Geometry: final body of the model. Coordinates: model frame, mm. A direction names the side the tool comes from. Round coordinates to 2 decimals unless told otherwise and drop trailing zeros. Write each loop counter-clockwise with the first axis right and the second up, starting at its lowest first coordinate (ties: lowest second). Pieces come first, ordered by that corner, then holes. Notation, with made-up numbers: (68, 85.25) -> (81, 85.25) arc R28 ccw to (81, 122.25) -> close; hole circle Ø5 at (44.25, 50). An arc over 180 degrees is marked (long way). One line per item, written item: value. Start each with the question number.
from build123d import *

# Parameters (mm, degrees)
F1_DEPTH = 10
F2_DEPTH = 85
F3_W     = 20
F3_H     = 25
F4_DEPTH = 88.4


with BuildPart() as f1:
    # F0 (on Top) → F1 (new body)
    with BuildSketch(Plane.XY):
        Polygon((-180, 30), (-180, 0), (0, 0), (0, 30), (-10, 30), (-10, 10), (-170, 10), (-170, 30), align=None)
    extrude(amount=F1_DEPTH)

    # F1_face (on face) → F2 (join)
    with BuildSketch(Plane(origin=(-90, 7.727273, 10), x_dir=(1, 0, 0), z_dir=(0, 0, 1))):
        Polygon((-90, 22.272727), (-90, -7.727273), (90, -7.727273), (90, 22.272727), (80, 22.272727), (80, 2.272727), (-80, 2.272727), (-80, 22.272727), align=None)
    extrude(amount=-F2_DEPTH)

    # F3 (on face) → F4 (cut)
    with BuildSketch(Plane.YZ):
        with Locations((20, -32.5)):
            Rectangle(F3_W, F3_H)
    extrude(amount=-F4_DEPTH, mode=Mode.SUBTRACT)


solid = f1.part
(1) Line query: probe 1 along X at (y, z) = (20.5, -63); probe 2 along Y at (x, z) = (-83, -63); probe 3 along X at (y, z) = (17, -38.5). Output: solid intervals per line, ascending.
(2) Section query A-A (y = 18.75). Output: boundary loops of the cut face in (x, z).
(3) Pull-direction query (Z, two-part tool) for faces 3 (the face through (-5, 20, -20)), 4 (the face through (-10, 20, -5)), 5 (the face through (-5, 20, -45)), 6 (the face through (-111, 9, 10)); classes: pulls with the +Z half, pulls with the -Z half, needs draft (parallel to the pull), parting line crosses it, or undercut.
(4) Section query C-C (x = -154.5). Output: boundary loops of the cut face in (y, z).
(5) Section query B-B (z = -49.5). Output: boundary loops of the cut face in (x, y).
(6) Set-up query: faces 1 (the face through (0, 8, -32)), 2 (the face through (-10, 20, -60)). Return all of +Z, -Z, +X, -X, +Y, -Y with unobstructed straight access to the full face (end or side cutting, diameter ignored); none if empty.
(7) Pin query (flat end, axial travel): pin 1 (2 mm diameter, centred on x = -83.5, z = -59.5, fed in from +Y). Return the tip coordinate at first contact, or that it passes through.
(8) Section query D-D (z = -31.5). Output: boundary loops of the cut face in (x, y), and give its area (3 significant figures).
Results list:
1. probe 1: x = -180 to -170, -10 to 0
1. probe 2: y = 0 to 10
1. probe 3: x = -180 to -170
2. outline: (-180, -75) -> (-170, -75) -> (-170, 10) -> (-180, 10) -> close; (-10, -75) -> (0, -75) -> (0, -45) -> (-10, -45) -> close; (-10, -20) -> (0, -20) -> (0, 10) -> (-10, 10) -> close
3. face 3: undercut
3. face 4: needs draft
3. face 5: undercut
3. face 6: pulls with the +Z half
4. outline: (0, -75) -> (10, -75) -> (10, 10) -> (0, 10) -> close
5. outline: (-180, 0) -> (0, 0) -> (0, 30) -> (-10, 30) -> (-10, 10) -> (-170, 10) -> (-170, 30) -> (-180, 30) -> close
6. face 1: +Z, -Z, +X, +Y, -Y
6. face 2: +Z, -Z, +Y
7. pin 1: stops at y = 10
8. outline: (-180, 0) -> (0, 0) -> (0, 10) -> (-170, 10) -> (-170, 30) -> (-180, 30) -> close
8. area: 2,000 mm^2
